Autodesk Inventor part; units mm, degrees
ref_plane "YZ Plane" through (0, 0, 0) normal (1, 0, 0) x (0, 1, 0)
ref_plane "XZ Plane" through (0, 0, 0) normal (0, 1, 0) x (-1, 0, 0)
ref_plane "XY Plane" through (0, 0, 0) normal (0, 0, 1) x (1, 0, 0)
sketch "Sketch1" plane through (0, 0, 0) normal (0, 0, 1) x (1, 0, 0)
  line L0 (0, 0) -> (400, 0)
  line L1 (400, 0) -> (400, 350)
  line L2 (400, 350) -> (0, 350)
  line L3 (0, 350) -> (0, 0)
  dimension "d0" = 400
  dimension "d1" = 350
extrude "Extrusion1" add sketch "Sketch1" along normal blind 20
sketch "Sketch2" plane through (0, 0, 0) normal (0, 0, -1) x (-1, 0, 0)
  circle A0 centre (-190.475, 175) radius 3
  circle A1 centre (-209.525, 175) radius 3
  point P0 (0, 0)
extrude "Extrusion2" cut sketch "Sketch2" against normal blind 20
sketch "Sketch4" plane through (0, 0, 0) normal (0, 0, -1) x (-1, 0, 0)
  circle A0 centre (-190.475, 175) radius 3 construction
  circle A1 centre (-209.525, 175) radius 3 construction
  circle A2 centre (-190.475, 175) radius 5
  circle A3 centre (-209.525, 175) radius 5
  point P0 (0, 0)
  dimension "d10" = 10
  dimension "d11" = 10
extrude "Extrusion4" cut sketch "Sketch4" against normal blind 6
equation "\"d0\" = maxl"
equation "\"d1\" = maxw"
equation "\"d2\" = platft"
equation "\"d4\" = platft"
equation "\"d10\" = bhd"
equation "\"d11\" = bhd"
equation "\"d12\" = bhh"
equation "\"dias\" = 8.8"
equation "\"stra1\" = 9.5"
equation "\"diab2\" = 6"
equation "\"stra\" = 25"
equation "\"db1\" = 6"
equation "\"ds1\" = 5.8"
equation "\"ds2\" = 1.6"
equation "\"ang\" = 120deg"
equation "\"db2\" = 3"
equation "\"diab3\" = 7"
equation "\"diab4\" = 3"
equation "\"dias1\" = 13.4375"
equation "\"dias3\" = 2"
equation "\"dias4\" = 4"
equation "\"t1\" = 3"
equation "\"t2\" = 3"
equation "\"t3\" = 6"
equation "\"t4\" = 6"
equation "\"t5\" = 3"
equation "\"diab1\" = 19"
equation "\"afw\" = 0.2"
equation "\"maxw\" = 350"
equation "\"lcsd\" = 19.05"
equation "\"lcwd1\" = 25"
equation "\"lch1\" = 39"
equation "\"lcwd2\" = 34"
equation "\"lcwd3\" = 43"
equation "\"dia1\" = 6"
equation "\"td\" = 18"
equation "\"bhh\" = 6"
equation "\"bhd\" = 10"
equation "\"spacert\" = 2"
equation "\"sh\" = 31"
equation "\"sw\" = 25"
equation "\"platft\" = 20"
equation "\"pvct\" = 5"
equation "\"dia3\" = 8"
equation "\"dia4\" = 11"
equation "\"tankl\" = 379"
equation "\"play\" = 9"
equation "\"holeh\" = 26"
equation "\"slack\" = 0.5"
equation "\"surroundt\" = 5"
equation "\"play2\" = 3"
equation "\"maxl\" = 400"
equation "\"diaoverflow\" = 25"
equation "\"diawater\" = 25"
equation "\"diacucl\" = 32"
equation "\"diaair\" = 32"
equation "\"diaph\" = 32"
equation "\"diasurroundhole\" = 42"
equation "\"diagrate\" = 12"
equation "\"gratespacing\" = 12.02082"
equation "\"sidedist\" = 13.9375"
equation "\"bottomdist\" = 9.6355"
equation "\"diahcl\" = 32"
equation "\"bracketwtop\" = 6"
equation "\"bracketwbottom\" = 6"
equation "\"nett\" = 1"
equation "\"nethole\" = 16"
equation "\"nettop\" = 7"
equation "\"netside\" = 3.5"
equation "\"netholespacing\" = 2"
equation "\"diaetape\" = 32"
properties part number "platform_top" material "PVC-Piping"
Input: part model. Units: mm. Frame: model coordinates. A direction names the side the tool comes from. Give positions to 0.01 mm unless a question says otherwise; leave off trailing zeros. One line per item, written item: value.
1. Pin query (flat end, axial travel): pin 1 Ø5 at (x, y) = (190.475, 175) entering from +Z. Return the tip coordinate at first contact, or that it passes through.
Determined:
pin 1: through
2. Reachability of faces 1 (the face through (203, 350, 10)), 2 (the face through (207, 173, 6)) from +Z, -Z, +X, -X, +Y, -Y: full face, straight path, thin tool, end or side. Return the list, or none.
Determined:
face 1: +Z, -Z, +X, -X, +Y
face 2: -Z
3. Line query: probe 1 along X at (y, z) = (175, 9) (3 decimals). Output: solid intervals per line, ascending.
Determined:
probe 1: 0 to 187.475, 193.475 to 206.525, 212.525 to 400
4. Draft query along X for faces 3 (the face through (206.84, 179.22, 2.96)), 4 (the face through (197, 177, 0)), 5 (the face through (0, 177, 10)). Return one class per face: released by +X, released by -X, zero draft, split by the parting line, or undercut.
Determined:
face 3: undercut
face 4: zero draft
face 5: released by -X
